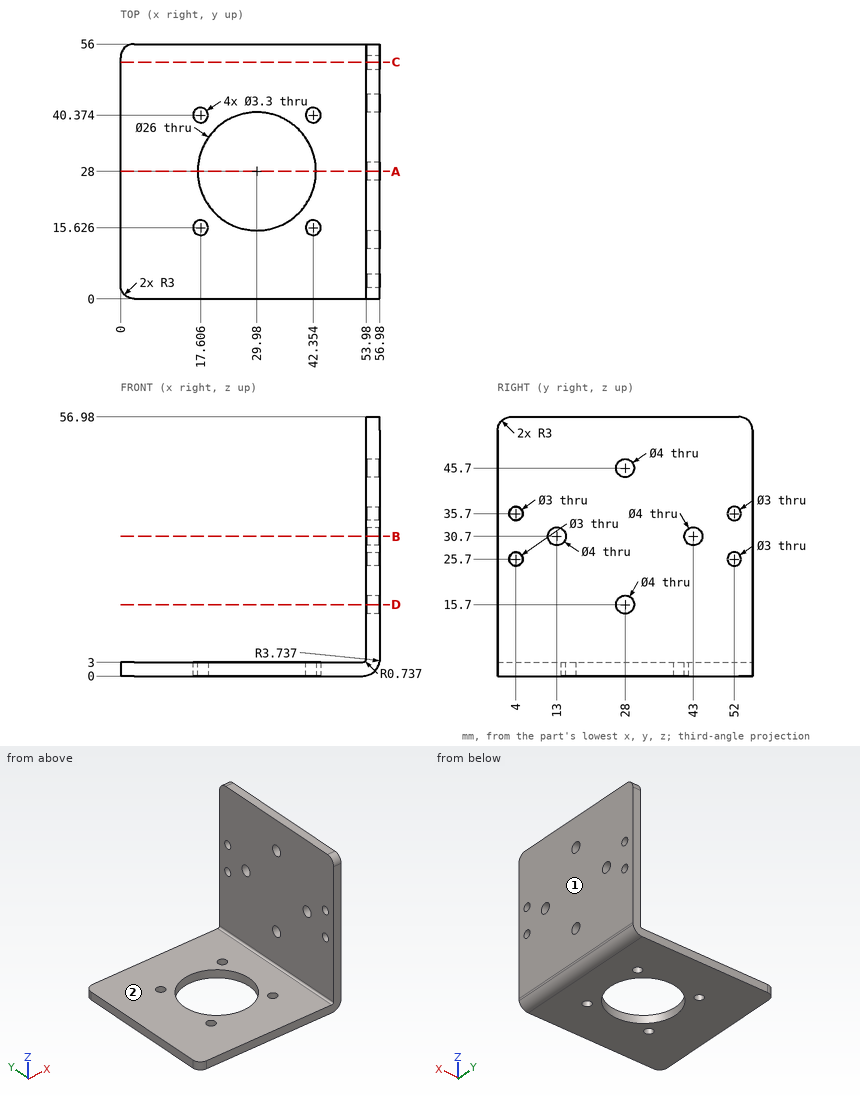
Check sheet for the drawn part. Datum: minimum x, y, z corner. Units: mm. A direction names the side the tool comes from. Coordinates: 2 decimals unless noted, no trailing zeros. Loops run counter-clockwise (first coordinate to the right, second up) from the corner with the lowest first, then second, coordinate; pieces in that order, holes last. Notation, with made-up numbers: (-1.75, 70) -> (13.25, 70) arc R23 cw to (13.25, 106) -> close; hole circle Ø4 at (84.25, 50.5). An arc over 180 degrees is marked (long way). Answer as a JSON object with one key per item and string values. Group by question number.
Item 1: Scan lines: probe 1 along X at (y, z) = (11.5, 15); probe 2 along Z at (x, y) = (8, 35); probe 3 along Y at (x, z) = (55.1, 45.7). Record each from-to range of solid material in increasing order.
Item 2: Sectioned sample at B-B on z = 30.7. Record the boundary of the cut face in (x, y), plus the area to 3 significant figures.
Item 3: Tool access check on the marked faces 1 and 2. Record the directions out of +Z, -Z, +X, -X, +Y, -Y that give a thin tool (end or side, any length) a straight path to the whole face; none if there is none.
Item 4: Depth check by flat-ended pin: pin 1 (16 mm diameter, centred on y = 37, z = 30.5, fed in from -X). Enter the tip coordinate at first touch or a pass-through.
Item 5: Sectioned sample at C-C on y = 52. Record the boundary of the cut face in (x, z), plus the area to 3 significant figures.
Item 6: Sectioned sample at D-D on z = 15.7. Record the boundary of the cut face in (x, y).
Item 7: Sectioned sample at A-A on y = 28. Record the boundary of the cut face in (x, z), plus the area to 3 significant figures.
Evaluation:
{
 "1": {"probe 1": "x = 53.98 to 56.98", "probe 2": "z = 0 to 3", "probe 3": "y = 0 to 26, 30 to 56"},
 "2": {"outline": "(53.98, 0) -> (56.98, 0) -> (56.98, 11) -> (53.98, 11) -> close; (53.98, 15) -> (56.98, 15) -> (56.98, 41) -> (53.98, 41) -> close; (53.98, 45) -> (56.98, 45) -> (56.98, 56) -> (53.98, 56) -> close", "area": "144 mm²"},
 "3": {"face 1": "+Z, -Z, +X, +Y, -Y", "face 2": "+Z, -X, +Y, -Y"},
 "4": {"pin 1": "stops at x = 53.98"},
 "5": {"outline": "(0, 0) -> (53.24, 0) arc R3.74 ccw to (56.98, 3.74) -> (56.98, 24.2) -> (53.98, 24.2) -> (53.98, 3.74) arc R0.74 cw to (53.24, 3) -> (0, 3) -> close; (53.98, 27.2) -> (56.98, 27.2) -> (56.98, 34.2) -> (53.98, 34.2) -> close; (53.98, 37.2) -> (56.98, 37.2) -> (56.98, 56.98) -> (53.98, 56.98) -> close", "area": "312 mm²"},
 "6": {"outline": "(53.98, 0) -> (56.98, 0) -> (56.98, 26) -> (53.98, 26) -> close; (53.98, 30) -> (56.98, 30) -> (56.98, 56) -> (53.98, 56) -> close"},
 "7": {"outline": "(0, 0) -> (16.98, 0) -> (16.98, 3) -> (0, 3) -> close; (42.98, 0) -> (53.24, 0) arc R3.74 ccw to (56.98, 3.74) -> (56.98, 13.7) -> (53.98, 13.7) -> (53.98, 3.74) arc R0.74 cw to (53.24, 3) -> (42.98, 3) -> close; (53.98, 17.7) -> (56.98, 17.7) -> (56.98, 43.7) -> (53.98, 43.7) -> close; (53.98, 47.7) -> (56.98, 47.7) -> (56.98, 56.98) -> (53.98, 56.98) -> close", "area": "228 mm²"}
}
